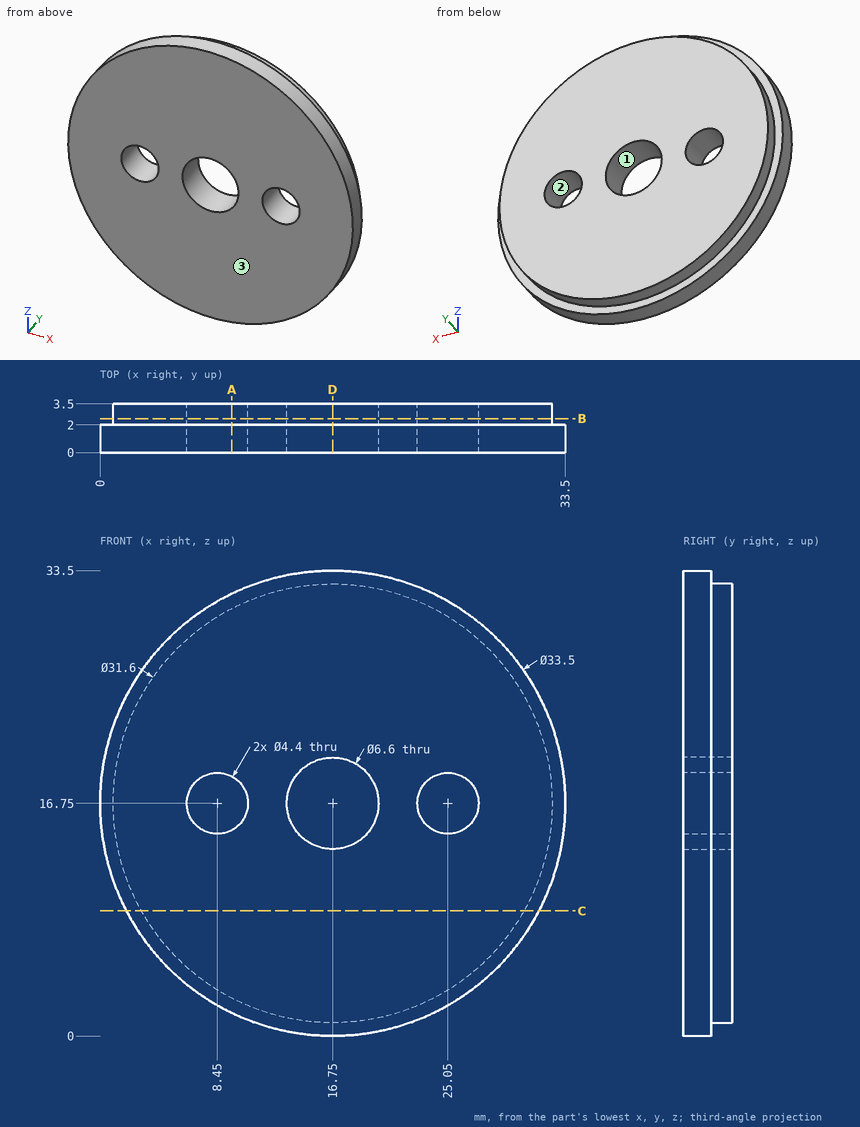
Design review of the part shown in the three views and the two pictorial views. Dimensions are in mm from the part's minimum x, y and z. Round coordinates to 2 decimals unless told otherwise and drop trailing zeros. Loops run counter-clockwise (first coordinate to the right, second up) from the corner with the lowest first, then second, coordinate; pieces in that order, holes last. Notation, with made-up numbers: M -18.5,-10 L 22.5,-10 A10 cw 22.5,5 Z; hole C -1.5,-22 d1. An arc over 180 degrees is marked long. Put each result on its own line as item: value.
Q1. To check wall thickness, follow L1, parallel to X at y = 1.15, z = 16.75; L2, parallel to X at y = 2.05, z = 16.75; L3, parallel to Y at x = 5.5, z = 28.5. State the ranges of each line that lie inside material, in increasing order.
Result set:
L1: x = 0 to 6.25, 10.65 to 13.45, 20.05 to 22.85, 27.25 to 33.5
L2: x = 0.95 to 6.25, 10.65 to 13.45, 20.05 to 22.85, 27.25 to 32.55
L3: y = 0 to 2
Q2. Consider section D-D, the plane x = 16.75. Give the boundary of the cut face in (y, z).
Result set:
outline: M 0,0 L 2,0 L 2,0.95 L 3.5,0.95 L 3.5,13.45 L 0,13.45 Z; M 0,20.05 L 3.5,20.05 L 3.5,32.55 L 2,32.55 L 2,33.5 L 0,33.5 Z
Q3. For pin 1 (8.5 mm diameter, centred on x = 16.75, z = 16.75, fed in from -Y); pin 2 (1 mm diameter, centred on y = 1.5, z = 7, fed in from -X), all flat-tipped, find the tip position at first contact; note any pin that passes through.
Result set:
pin 1: stops at y = 0
pin 2: stops at x = 2.79
Q4. Consider section A-A, the plane x = 9.5. Give the boundary of the cut face in (y, z).
Result set:
outline: M 0,1.65 L 2,1.65 L 2,2.71 L 3.5,2.71 L 3.5,14.82 L 0,14.82 Z; M 0,18.68 L 3.5,18.68 L 3.5,30.79 L 2,30.79 L 2,31.85 L 0,31.85 Z
Q5. Consider section B-B, the plane y = 2.45. Give the boundary of the cut face in (x, z), then the cut area to 3 significant figures.
Result set:
outline: C 16.75,16.75 d31.6; hole C 8.45,16.75 d4.4; hole C 16.75,16.75 d6.6; hole C 25.05,16.75 d4.4
area: 720 mm²
Q6. Mouldability with a two-part tool opening along Z and no side actions: class the marked faces 1, 2 and 3 as released by +Z, released by -Z, zero draft, split by the parting line, or undercut.
Result set:
face 1: undercut
face 2: undercut
face 3: zero draft
Q7. Consider section C-C, the plane z = 9. Give the boundary of the cut face in (x, y).
Result set:
outline: M 1.9,0 L 31.6,0 L 31.6,2 L 30.52,2 L 30.52,3.5 L 2.98,3.5 L 2.98,2 L 1.9,2 Z
